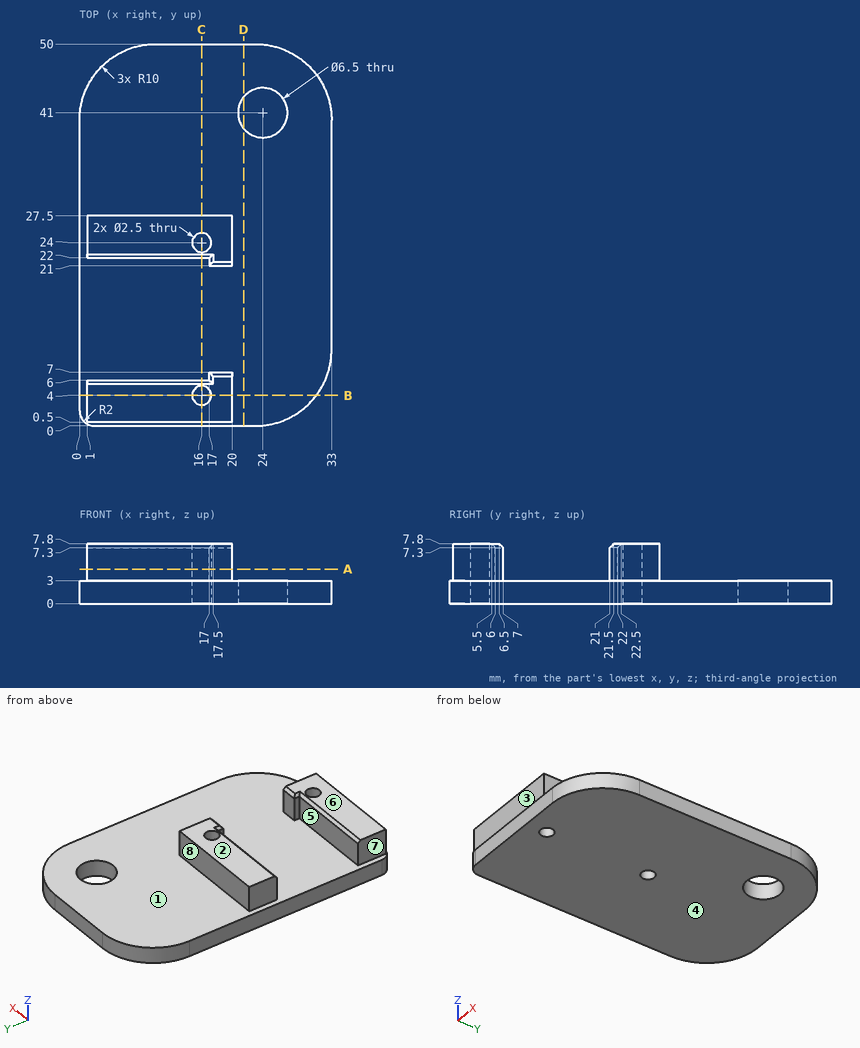
Source: three-view drawing plus pictorial views. Frame: mm from the lowest corner of the part. A direction names the side the tool comes from. Give positions to 0.01 mm unless a question says otherwise; leave off trailing zeros. Order: outer loops, then holes, each group sorted by start corner. A loop starts at its lowest first (then second) coordinate and runs counter-clockwise, first axis right, second up. Notation, with made-up numbers: M -17.5,12.5 L 14.5,12.5 A23 cw 14.5,39.5 Z; hole C 65,73 d2. An arc over 180 degrees is marked long. Return JSON: item names as keys, results as strings.
1) Line query: L1, parallel to Y at x = 16, z = 4; L2, parallel to Y at x = 6, z = 3.25; L3, parallel to Y at x = 15, z = 2.25. Output: solid intervals per line, ascending. Write a range as [from, to].
Taken from the geometry:
{"L1": "y = [0.5, 2.75], [5.25, 6], [22, 22.75], [25.25, 27.5]", "L2": "y = [0.5, 6], [22, 27.5]", "L3": "y = [0, 3.25], [4.75, 23.25], [24.75, 50]"}
2) Section query A-A on z = 4.5. Output: boundary loops of the cut face in (x, y).
Taken from the geometry:
{"outline": "M 1,0.5 L 20,0.5 L 20,7 L 17,7 L 17,6 L 1,6 Z; M 1,22 L 17,22 L 17,21 L 20,21 L 20,27.5 L 1,27.5 Z; hole C 16,4 d2.5; hole C 16,24 d2.5"}
3) Section query B-B on y = 4. Output: boundary loops of the cut face in (x, z).
Taken from the geometry:
{"outline": "M 0,0 L 14.75,0 L 14.75,7.8 L 1,7.8 L 1,3 L 0,3 Z; M 17.25,0 L 31,0 L 31,3 L 20,3 L 20,7.8 L 17.25,7.8 Z"}
4) Contact query for flat-ended pins moving along their axis: pin 1 (2.5 mm diameter, centred on x = 19, z = 5, fed in from +Y); pin 2 (0.5 mm diameter, centred on y = 21.5, z = 4.5, fed in from -X); pin 3 (1.1 mm diameter, centred on y = 6.5, z = 5, fed in from -X). Output: stop coordinate, or through.
Taken from the geometry:
{"pin 1": "stops at y = 27.5", "pin 2": "stops at x = 17", "pin 3": "stops at x = 1"}
5) Mould query, pull axis Y, two halves, no side actions, for the marked faces 1, 2 and 3. Classes: released by +Y, released by -Y, zero draft, split by the parting line, or undercut.
Taken from the geometry:
{"face 1": "undercut", "face 2": "zero draft", "face 3": "released by -Y"}
6) Section query D-D on x = 21.5. Output: boundary loops of the cut face in (y, z), and give its area (3 significant figures).
Taken from the geometry:
{"outline": "M 0,0 L 38.92,0 L 38.92,3 L 0,3 Z; M 43.08,0 L 50,0 L 50,3 L 43.08,3 Z", "area": "138 mm2"}
7) Section query C-C on x = 16. Output: boundary loops of the cut face in (y, z), and give its area (3 significant figures).
Taken from the geometry:
{"outline": "M 0,0 L 2.75,0 L 2.75,7.8 L 0.5,7.8 L 0.5,3 L 0,3 Z; M 5.25,0 L 22.75,0 L 22.75,7.8 L 22.5,7.8 L 22,7.3 L 22,3 L 6,3 L 6,7.3 L 5.5,7.8 L 5.25,7.8 Z; M 25.25,0 L 50,0 L 50,3 L 27.5,3 L 27.5,7.8 L 25.25,7.8 Z", "area": "164 mm2"}
8) Access query for the marked faces 4, 5, 6, 7 and 8. Directions: +Z, -Z, +X, -X, +Y, -Y. A direction counts if a zero-diameter tool reaches every point of the face in a straight line with its end or side. Return the directions, or none.
Taken from the geometry:
{"face 4": "-Z, +X, -X, +Y, -Y", "face 5": "+Z, -X", "face 6": "+Z, +X, -X, +Y, -Y", "face 7": "+Z, -X, +Y, -Y", "face 8": "+Z, +X, -X, +Y"}
